Autodesk Inventor part; units mm, degrees
ref_plane "YZ Plane" through (0, 0, 0) normal (1, 0, 0) x (0, 1, 0)
ref_plane "XZ Plane" through (0, 0, 0) normal (0, 1, 0) x (-1, 0, 0)
ref_plane "XY Plane" through (0, 0, 0) normal (0, 0, 1) x (1, 0, 0)
sketch "Sketch1" plane through (0, 0, 0) normal (0, 0, 1) x (1, 0, 0)
  line L0 (3, 12) -> (14, 12)
  line L1 (14, 12) -> (14, 0)
  line L2 (3, 2) -> (3, 12)
  line L3 (0, 19.5472) -> (0, -22.4151)
  line L4 (14, 0) -> (13, 0) construction
  line L5 (13, 0) -> (13, -6)
  line L6 (13, -6) -> (14, -6)
  line L7 (14, -6) -> (14, 0)
  line L8 (11.4, 0) -> (10.4, 0) construction
  line L9 (10.4, 0) -> (10.4, -6) construction
  line L10 (10.4, -6) -> (11.4, -6) construction
  line L11 (11.4, -6) -> (11.4, 0)
  line L12 (11.4, -6) -> (11.4, -12)
  line L13 (11.4, -12) -> (11.3, -12)
  line L14 (11.3, -12) -> (10.4892, -6.5945)
  arc A0 (3, 2) -> (4.4967, 0.0644) centre (5, 2) ccw
  line L15 (13, 0) -> (11.4, 0)
  line L16 (10.4, 0) -> (5, 0)
  line L17 (-20.0393, 0) -> (13, 0) construction
  line L18 (14, 0) -> (24.5476, 0) construction
  line L19 (5.48, -0.5334) -> (9.9979, -5.5532)
  arc A1 (10.4892, -6.5945) -> (9.9979, -5.5532) centre (8.5113, -6.8911) ccw
  arc A2 (5.48, -0.5334) -> (4.4967, 0.0644) centre (3.9934, -1.8713) ccw
  point P0 (0, 0)
  point P1 (10.4, 0)
  point P2 (10.5, -6)
  dimension "d0" = 6
  dimension "d2" = 1
  dimension "d4" = 1
  dimension "d5" = 6
  dimension "d6" = 1.6
  dimension "d7" = 26
  dimension "d9" = 6
  dimension "d10" = 0.1
  dimension "d11" = 2
  dimension "d12" = 12
  dimension "d14" = 6
  dimension "d41" = 2
  dimension "d42" = 2
revolve "Revolution1" add sketch "Sketch1" angle 360 about axis through (0, 19.5472, 0) along (0, -1, 0)
sketch "Sketch2" plane through (0, 0, 0) normal (0, 0, 1) x (1, 0, 0)
  line L0 (-3, 12) -> (3, 12)
  line L1 (0, 12) -> (0, 0) construction
  line L2 (-3, 2) -> (3, 2) construction
  circle A0 centre (0, 3.5) radius 3
  line L3 (-13, 0) -> (13, 0) construction
  point P0 (2.5981, 2)
  point P1 (-2.5981, 2)
  dimension "d16" = 6
  dimension "d43" = 3.5
extrude "Extrusion1" cut sketch "Sketch2" along normal blind 3 and the other way blind 19.5
sketch "Sketch4" plane through (0, 12, 0) normal (0, 1, 0) x (1, 0, 0)
  circle A0 centre (0, 0) radius 6.6
  dimension "d38" = 13.2
extrude "Extrusion3" cut sketch "Sketch4" against normal blind 5
sketch "Sketch3" plane through (0, 12, 0) normal (0, 1, 0) x (1, 0, 0)
  circle A0 centre (-5.25, 0) radius 0.45
  line L0 (0, 0) -> (-14, 0) construction
  circle A1 centre (0, 0) radius 14 construction
  circle A2 centre (-7.5, 0) radius 0.45
  circle A3 centre (0, 0) radius 3 construction
  arc A4 (-2.5981, 1.5) -> (-2.5981, -1.5) centre (0, 0) ccw construction
  circle A5 centre (-6.4952, -3.75) radius 0.45
  circle A6 centre (-4.5466, -2.625) radius 0.45
  circle A7 centre (-3.75, -6.4952) radius 0.45
  circle A8 centre (-2.625, -4.5466) radius 0.45
  circle A9 centre (0, -7.5) radius 0.45
  circle A10 centre (0, -5.25) radius 0.45
  circle A11 centre (3.75, -6.4952) radius 0.45
  circle A12 centre (2.625, -4.5466) radius 0.45
  circle A13 centre (6.4952, -3.75) radius 0.45
  circle A14 centre (4.5466, -2.625) radius 0.45
  circle A15 centre (7.5, 0) radius 0.45
  circle A16 centre (5.25, 0) radius 0.45
  circle A17 centre (6.4952, 3.75) radius 0.45
  circle A18 centre (4.5466, 2.625) radius 0.45
  circle A19 centre (3.75, 6.4952) radius 0.45
  circle A20 centre (2.625, 4.5466) radius 0.45
  circle A21 centre (0, 7.5) radius 0.45
  circle A22 centre (0, 5.25) radius 0.45
  circle A23 centre (-3.75, 6.4952) radius 0.45
  circle A24 centre (-2.625, 4.5466) radius 0.45
  circle A25 centre (-6.4952, 3.75) radius 0.45
  circle A26 centre (-4.5466, 2.625) radius 0.45
  point P0 (-3, 0)
  point P1 (-3, 0)
  dimension "d22" = 0.9
  dimension "d24" = 0.9
  dimension "d30" = 2.25
  dimension "d31" = 2.25
  dimension "d34" = 360
equation "\"d0\" = t_D"
equation "\"d2\" = w_th"
equation "\"d4\" = w_th"
equation "\"d5\" = w_l"
equation "\"d6\" = lv_th"
equation "\"d7\" = lv_OD"
equation "\"d9\" = w_l"
equation "\"d10\" = tol"
equation "\"d11\" = fillet_D"
equation "\"d12\" = top_th_f"
equation "\"d14\" = w_l"
equation "\"d41\" = fillet_D"
equation "\"d42\" = fillet_D"
equation "\"d16\" = t_D"
equation "\"d43\" = 0.5 * w_th + 0.5 * t_D"
equation "\"d18\" = 0.5 * t_D"
equation "\"d19\" = 0.75 * lv_OD"
equation "\"d38\" = cn_D"
equation "\"d39\" = cn_h"
equation "\"d22\" = h_D"
equation "\"d24\" = h_D"
equation "\"d30\" = h_s"
equation "\"tol\" = 0.1"
equation "\"fillet_D\" = 2"
equation "\"w_th\" = 1"
equation "\"w_l\" = 6"
equation "\"t_D\" = 6"
equation "\"t_D_f\" = t_D + w_th"
equation "\"top_th_f\" = t_D_f + cn_h"
equation "\"cn_h\" = 5"
equation "\"lv_OD\" = 26"
equation "\"lv_th\" = 1.6"
equation "\"d3\" = w_l"
equation "\"d8\" = top_th_f"
equation "\"top_th\" = t_D + w_th"
equation "\"sv_OD\" = 13"
equation "\"sv_th\" = 1.5"
equation "\"b_OD\" = 44"
equation "\"b_th\" = 1.5"
equation "\"b_ID\" = 36.5"
equation "\"b_rim_h\" = 5"
equation "\"h_s\" = 2.25"
equation "\"h_D\" = 0.9"
equation "\"d25\" = 2 * d26"
equation "\"v_h_D\" = 7.5"
equation "\"v_h_off\" = 0.5 * cn_D + 0.5 * v_h_D"
properties part number "vial"
Check sheet for the modelled part. Datum: model origin and axes. Units: mm. A direction names the side the tool comes from. Round coordinates to 2 decimals unless told otherwise and drop trailing zeros. Write each loop counter-clockwise with the first axis right and the second up, starting at its lowest first coordinate (ties: lowest second). Pieces come first, ordered by that corner, then holes. Notation, with made-up numbers: (66.25, -3.75) - (94.25, -3.75) arc R13 cw to (94.25, 21.25) - close; hole circle Ø2 at (20, 34). An arc over 180 degrees is marked (long way). Return JSON: item names as keys, results as strings.
Q1. Cross-section at A-A (z = -12.5). Record the boundary of the cut face in (x, y).
Returned:
{"outline": "(-6.3, -6) - (-3.57, -6) - (-3.57, 0) - (3.57, 0) - (3.57, -6) - (6.3, -6) - (6.3, 12) - (-6.3, 12) - close; hole circle Ø6 at (0, 3.5)"}
Q2. Scan lines: L1, parallel to Z at x = -10.25, y = -3; L2, parallel to Z at x = -3.75, y = -2.5; L3, parallel to Z at x = 0, y = 9.7. Record each from-to range of solid material in increasing order. Write a range as from..to.
Returned:
{"L1": "z = -9.54..-8, -4.99..4.99, 8..9.54", "L2": "z = -13.49..-12.45, -10.77..-6.2, 6.2..10.77, 12.45..13.49", "L3": "z = -14..-6.6, 6.6..14"}
Q3. Cross-section at D-D (y = 3). Record the boundary of the cut face in (x, z), then the cut area to 3 significant figures.
Returned:
{"outline": "(-2.96, -13.68) - (-2.96, -0.5) arc R3 cw to (-2.96, 0.5) - (-2.96, 3) - (2.96, 3) - (2.96, 0.5) arc R3 cw to (2.96, -0.5) - (2.96, -13.68) arc R14 ccw (long way) to start", "area": "516 mm²"}
Q4. Access from +Z, -Z, +X, -X, +Y, -Y to the whole of each face (thin tool, end or side, straight path). Record for faces 5 (the cylindrical face through (-10.316, -3.042, -7.91)), 6 (the cylindrical face through (-2.995, 3.336, 2.146)), 7 (the cylindrical face through (3, 3, 0)).
Returned:
{"face 5": "-Y", "face 6": "-Z", "face 7": "+Y, -Y"}
Q5. Depth check by flat-ended pin: P1, Ø2, axis at y = 1, z = 5, coming from the -X side; P2, Ø8, axis at x = 9, y = 6, coming from the -Z side; P3, Ø1, axis at y = 1, z = -9, coming from the -X side; P4, Ø5.5, axis at x = 0, z = 0, coming from the -Y side. Enter the tip coordinate at first touch or a pass-through.
Returned:
{"P1": "stops at x = -13.42", "P2": "stops at z = -13.08", "P3": "stops at x = -11.12", "P4": "passes through"}
Q6. Cross-section at B-B (y = -3.5). Record the boundary of the cut face in (x, z).
Returned:
{"outline": "circle Ø28 at (0, 0); circle Ø22.8 at (0, 0); hole circle Ø26 at (0, 0); hole circle Ø16.3 at (0, 0)"}
Q7. Draft check along Y on faces 1 (the cylindrical face through (-9, -6, 7)), 2 (the conical face through (-1.25, -0.85, -5.63)), 3 (the cylindrical face through (3, 3.4, 2.1)), 4 (the flat face through (6, 12, 3.3)). Enter one of: released by +Y, released by -Y, zero draft, split by the parting line, or undercut.
Returned:
{"face 1": "zero draft", "face 2": "released by -Y", "face 3": "undercut", "face 4": "released by +Y"}
